from build123d import *

# Parameters (mm, degrees)
SKETCH1_R           = 1.9
BOSS_EXTRUDE1_DEPTH = 4


with BuildPart() as part:
    # Sketch1 → Boss-Extrude1 (new body)
    with BuildSketch(Plane.XY):
        with BuildLine():
            Line((17.801991214, -63.605751381), (15.909561323, -56.844180516))
            ThreePointArc((15.909561323, -56.844180516), (17.331888256, -53.097314134), (21.331580773, -53.351245934))
            ThreePointArc((21.331580773, -53.351245934), (25.046699576, -54.90531314), (28.9855978, -54.067271739))
            ThreePointArc((28.9855978, -54.067271739), (0, 56.55), (-28.9855978, -54.067271739))
            ThreePointArc((-28.9855978, -54.067271739), (-25.046699576, -54.90531314), (-21.331580773, -53.351245934))
            ThreePointArc((-21.331580773, -53.351245934), (-17.331888256, -53.097314134), (-15.909561323, -56.844180516))
            Line((-15.909561323, -56.844180516), (-17.801991214, -63.605751381))
            ThreePointArc((-17.801991214, -63.605751381), (0, 66.05), (17.801991214, -63.605751381))
        make_face()
        with Locations((19.159665955, -55.934540541)):
            Circle(SKETCH1_R, mode=Mode.SUBTRACT)
        with Locations((-19.159665955, -55.934540541)):
            Circle(SKETCH1_R, mode=Mode.SUBTRACT)
    extrude(amount=BOSS_EXTRUDE1_DEPTH)


solid = part.part
Geometry check sheet. Reference: the model listing, model coordinates, mm. A direction names the side the tool comes from. Round coordinates to 2 decimals unless told otherwise and drop trailing zeros. Loops run counter-clockwise (first coordinate to the right, second up) from the corner with the lowest first, then second, coordinate; pieces in that order, holes last. Notation, with made-up numbers: (14, 80) - (51, 80) arc R22 cw to (51, 98) - close; hole circle Ø11 at (42.5, -16.5). An arc over 180 degrees is marked (long way). Answer as CSV lines item,"result".
(1) Depth check by flat-ended pin: pin 1 Ø2 at (y, z) = (38, 2.5) entering from -X. Enter the tip coordinate at first touch or a pass-through.
Output values:
pin 1,"stops at x = -54.71"
(2) Cross-section at C-C, the plane z = 3.2. Enter the section's corners in (x, y) (3 decimals), and give its area (3 significant figures).
Output values:
outline,"(-28.986, -54.067) arc R59.106 cw (long way) to (28.986, -54.067) arc R6.75 cw to (21.332, -53.351) arc R3.375 ccw to (15.91, -56.844) - (17.802, -63.606) arc R66.05 ccw (long way) to (-17.802, -63.606) - (-15.91, -56.844) arc R3.375 ccw to (-21.332, -53.351) arc R6.75 cw to start; hole circle Ø3.8 at (-19.16, -55.935); hole circle Ø3.8 at (19.16, -55.935)"
area,"2,630 mm²"
(3) Release check for a two-part mould opening along X. For faces 4 (the face through (17.28, -53.13, 1.97)), 5 (the face through (20, 54, 4)), 6 (the face through (-2.652, 65.997, 1.972)), 7 (the face through (-17.35, -55.36, 1.97)) record: released by +X, released by -X, zero draft, split by the parting line, or undercut.
Output values:
face 4,"undercut"
face 5,"zero draft"
face 6,"split by the parting line"
face 7,"undercut"
(4) Set-up check for faces 1 (the face through (-25.1, -54.91, 1.97)), 2 (the face through (20, 54, 0)), 3 (the face through (-16.843, -60.178, 1.972)): record each of +Z, -Z, +X, -X, +Y, -Y from which the full face is reachable in a straight line by a thin tool's end or side.
Output values:
face 1,"+Z, -Z"
face 2,"-Z, +X, -X, +Y, -Y"
face 3,"+Z, -Z, -Y"
(5) Material ranges on line 1 along X through (y, z) = (-1, 2.7); line 2 along Y through (x, z) = (-41.5, 1.1); line 3 along X through (y, z) = (-15, 1.15), recorded low to high.
Output values:
line 1,"x = -66.04 to -59.09, 59.09 to 66.04"
line 2,"y = -51.38 to -44.64, 39.53 to 51.38"
line 3,"x = -64.32 to -57.78, 57.78 to 64.32"
(6) Cross-section at D-D, the plane x = 0. Enter the section's corners in (y, z), and give its area (3 significant figures).
Output values:
outline,"(56.55, 0) - (66.05, 0) - (66.05, 4) - (56.55, 4) - close"
area,"38.0 mm²"
(7) Cross-section at B-B, the plane y = -6. Enter the section's corners in (x, z).
Output values:
outline,"(-65.78, 0) - (-59.01, 0) - (-59.01, 4) - (-65.78, 4) - close; (59.01, 0) - (65.78, 0) - (65.78, 4) - (59.01, 4) - close"
(8) Cross-section at A-A, the plane x = 27.5. Enter the section's corners in (y, z), and give its area (3 significant figures).
Output values:
outline,"(-60.05, 0) - (-54.68, 0) - (-54.68, 4) - (-60.05, 4) - close; (49.76, 0) - (60.05, 0) - (60.05, 4) - (49.76, 4) - close"
area,"62.6 mm²"
